Could you check a few things on this model? Use its own coordinates, in mm. A direction names the side the tool comes from. Give positions to 0.01 mm unless a question says otherwise; leave off trailing zeros. Loops run counter-clockwise (first coordinate to the right, second up) from the corner with the lowest first, then second, coordinate; pieces in that order, holes last. Notation, with made-up numbers: M 34,21.25 L 70,21.25 A19 cw 70,57.25 Z; hole C 50,9 d5. An arc over 180 degrees is marked long. Use CSV: the item, a comma, the result in double quotes.
```python
from build123d import *

# Parameters (mm, degrees)
BOSS_EXTRU_1_DEPTH      = 10.5
ENL_V_MAT_EXTRU_1_DEPTH = 6.5
ESQUISSE3_R             = 4
ENL_V_MAT_EXTRU_2_DEPTH = 27.272609311
CONG_1_R                = 2


with BuildPart() as part:
    # Esquisse1 → Boss.-Extru.1 (new body)
    with BuildSketch(Plane(origin=(0, 0, 0), x_dir=(1, 0, 0), z_dir=(0, 1, 0))):
        with BuildLine():
            Line((0, 18), (16, 18))
            Line((16, 18), (16, -18))
            Line((16, -18), (0, -18))
            ThreePointArc((0, -18), (-18, 0), (0, 18))
        make_face()
    extrude(amount=BOSS_EXTRU_1_DEPTH)

    # Esquisse2 → Enlèv. mat.-Extru.1 (cut)
    with BuildSketch(Plane(origin=(0, 0, 0), x_dir=(1, 0, 0), z_dir=(0, 1, 0))):
        Polygon((0, -7.505553499), (6.5, -3.75277675), (6.5, 3.75277675), (0, 7.505553499), (-6.5, 3.75277675), (-6.5, -3.75277675), align=None)
    extrude(amount=ENL_V_MAT_EXTRU_1_DEPTH, mode=Mode.SUBTRACT)

    # Esquisse3 → Enlèv. mat.-Extru.2 (cut, through all)
    with BuildSketch(Plane(origin=(0, 6.5, 0), x_dir=(-1, 0, 0), z_dir=(0, -1, 0))):
        with Locations(Location((0, 0, 0), (0, 0, 90))):
            Circle(ESQUISSE3_R)
    extrude(amount=-ENL_V_MAT_EXTRU_2_DEPTH, mode=Mode.SUBTRACT)

    # Congé1
    cong_1_edges = [part.edges().sort_by_distance(p)[0] for p in [
        (8, 10.5, -18),
        (-18, 10.5, 0),
        (16, 0, 0),
        (8, 10.5, 18),
    ]]
    fillet(cong_1_edges, radius=CONG_1_R)


solid = part.part
```
1. I want a section at A-A, the plane z = 0. List the corners of the cut face in (x, y) for me.
Outcome:
outline,"M -18,0 L -6.5,0 L -6.5,6.5 L -4,6.5 L -4,10.5 L -16,10.5 A2 ccw -18,8.5 Z; M 4,6.5 L 6.5,6.5 L 6.5,0 L 14,0 A2 ccw 16,2 L 16,10.5 L 4,10.5 Z"
2. Please list where these lines run through material, in increasing order: line 1 (X direction, y = 8.2, z = 0); line 2 (Y direction, x = 0.5, z = -5); line 3 (Z direction, x = -5, y = 6.25).
Outcome:
line 1,"-18 to -4, 4 to 16"
line 2,"6.5 to 10.5"
line 3,"-17.29 to -4.62, 4.62 to 17.29"
3. I want a section at B-B, the plane x = 2. List the corners of the cut face in (y, z) for me.
Outcome:
outline,"M 0,-18 L 8.5,-18 A2 ccw 10.5,-16 L 10.5,-3.46 L 6.5,-3.46 L 6.5,-6.35 L 0,-6.35 Z; M 0,6.35 L 6.5,6.35 L 6.5,3.46 L 10.5,3.46 L 10.5,16 A2 ccw 8.5,18 L 0,18 Z"
4. I'm going to push a flat-ended pin straight in: pin 1 Ø2 at (y, z) = (4.5, -0.5) entering from -X. Where does the tip first touch, or does it pass through?
Outcome:
pin 1,"x = -18"
5. If we mould it in two halves opening along X, with no side actions, what happens to faces 3 (the face through (3.2, 3.2, 5.66)), 4 (the face through (15.43, 0.6, 0.25)), 5 (the face through (4, 10.5, 3))? For each: +X half, -X half, draft (parallel to the pull), parting line (faces both ways), or undercut.
Outcome:
face 3,"undercut"
face 4,"+X half"
face 5,"draft"
6. Which directions (+Z, -Z, +X, -X, +Y, -Y) give clear straight access to the entire face, cutting with the end or side of a thin tool? Please do faces 1 (the face through (-3.905, 8.472, 0.867)), 2 (the face through (-3.2, 3.2, -5.66)).
Outcome:
face 1,"+Y, -Y"
face 2,"-Y"
7. I want a section at C-C, the plane y = 5.25. List the corners of the cut face in (x, z) for me, then the cut area to 3 significant figures.
Outcome:
outline,"M 0,-18 L 16,-18 L 16,18 L 0,18 A18 ccw Z; hole M -6.5,-3.75 L 0,-7.51 L 6.5,-3.75 L 6.5,3.75 L 0,7.51 L -6.5,3.75 Z"
area,"939 mm2"
